Geometry check sheet. Reference: the model listing, model coordinates, mm. A direction names the side the tool comes from. Round coordinates to 2 decimals unless told otherwise and drop trailing zeros. Loops run counter-clockwise (first coordinate to the right, second up) from the corner with the lowest first, then second, coordinate; pieces in that order, holes last. Notation, with made-up numbers: (64, 45) - (111, 45) arc R8 cw to (111, 57) - close; hole circle Ø9 at (82, 41). An arc over 180 degrees is marked (long way). Answer as CSV lines item,"result". Start each with the question number.
1) Cross-section at A-A on z = 2.75. Record the boundary of the cut face in (x, y).
2) Cross-section at C-C on z = -0.5. Record the boundary of the cut face in (x, y) (3 decimals).
3) Cross-section at B-B on x = 0. Record the boundary of the cut face in (y, z), and give its area (3 significant figures).
4) Thickness scan on line 1 along Y through (x, z) = (0, 1.1); line 2 along Z through (x, y) = (9.75, -5.75); line 3 along X through (y, z) = (-5.5, -2.5). Record the ranges inside material, lowest first.
5) Draft check along Y on faces 1 (the cylindrical face through (-8.21, 8.65, 1.88)), 2 (the flat face through (0, -10.16, -2)), 3 (the cylindrical face through (-5.08, -0.13, 1.5)). Enter one of: released by +Y, released by -Y, zero draft, split by the parting line, or undercut.
6) Depth check by flat-ended pin: P1, Ø3, axis at x = -1.5, y = -2, coming from the +Z side. Enter the tip coordinate at first touch or a pass-through.
7) Cross-section at D-D on y = 0. Record the boundary of the cut face in (x, z).
8) Access from +Z, -Z, +X, -X, +Y, -Y to the whole of each face (thin tool, end or side, straight path). Record for faces 4 (the cylindrical face through (10.882, -0.101, -1.503)), 5 (the cylindrical face through (7.034, -6.493, 1.878)).
from build123d import *

# Parameters (mm, degrees)
BOSS_EXTRUDE5_DEPTH = 3.048
BOSS_EXTRUDE6_DEPTH = 3.048
PRONGS_R            = 1.27
BOSS_EXTRUDE7_DEPTH = 3.81


with BuildPart() as part:
    # Back Plate → Boss-Extrude5 (new body)
    with BuildSketch(Plane.XY):
        with BuildLine():
            Line((0, -10.16), (7.62, -10.16))
            ThreePointArc((7.62, -10.16), (9.416051224, -9.416051224), (10.16, -7.62))
            ThreePointArc((10.16, -7.62), (9.867513929, -5.715), (10.16, -3.81))
            ThreePointArc((10.16, -3.81), (10.882617987, -0.046833682), (10.16, 3.716332637))
            ThreePointArc((10.16, 3.716332637), (9.867513929, 5.621332637), (10.16, 7.526332637))
            ThreePointArc((10.16, 7.526332637), (9.416051224, 9.322383861), (7.62, 10.066332637))
            Line((7.62, 10.066332637), (-7.62, 10.066332637))
            ThreePointArc((-7.62, 10.066332637), (-9.416051224, 9.322383861), (-10.16, 7.526332637))
            ThreePointArc((-10.16, 7.526332637), (-9.867513929, 5.621332637), (-10.16, 3.716332637))
            ThreePointArc((-10.16, 3.716332637), (-10.882617987, -0.046833682), (-10.16, -3.81))
            ThreePointArc((-10.16, -3.81), (-9.867513929, -5.715), (-10.16, -7.62))
            ThreePointArc((-10.16, -7.62), (-9.416051224, -9.416051224), (-7.62, -10.16))
            Line((-7.62, -10.16), (0, -10.16))
        make_face()
    extrude(amount=-BOSS_EXTRUDE5_DEPTH)

    # Inner Circle → Boss-Extrude6 (add)
    with BuildSketch(Plane.XY):
        with BuildLine():
            Line((3.624386403, 3.559525699), (3.984498069, 3.917846237))
            ThreePointArc((3.984498069, 3.917846237), (-5.58790138, 0.033198873), (3.937664969, -3.96491344))
            Line((3.937664969, -3.96491344), (3.577553303, -3.606592902))
            ThreePointArc((3.577553303, -3.606592902), (-5.079891518, 0.033198873), (3.624386403, 3.559525699))
        make_face()
    extrude(amount=BOSS_EXTRUDE6_DEPTH)

    # Prongs → Boss-Extrude7 (add)
    with BuildSketch(Plane.XY):
        with Locations(Location((-7.62, 7.526332637, 0), (0, 0, 180))):
            Circle(PRONGS_R)
        with Locations(Location((7.62, -7.62, 0), (0, 0, 180))):
            Circle(PRONGS_R)
    extrude(amount=BOSS_EXTRUDE7_DEPTH)


solid = part.part
Answer block:
1,outline,"circle Ø2.54 at (-7.62, 7.53); (3.58, -3.61) arc R5.08 cw (long way) to (3.62, 3.56) - (3.98, 3.92) arc R5.59 ccw (long way) to (3.94, -3.96) - close; circle Ø2.54 at (7.62, -7.62)"
2,outline,"(-10.16, -7.62) arc R2.54 ccw to (-7.62, -10.16) - (7.62, -10.16) arc R2.54 ccw to (10.16, -7.62) arc R6.35 cw to (10.16, -3.81) arc R10.16 ccw to (10.16, 3.716) arc R6.35 cw to (10.16, 7.526) arc R2.54 ccw to (7.62, 10.066) - (-7.62, 10.066) arc R2.54 ccw to (-10.16, 7.526) arc R6.35 cw to (-10.16, 3.716) arc R10.16 ccw to (-10.16, -3.81) arc R6.35 cw to start"
3,outline,"(-10.16, -3.05) - (10.07, -3.05) - (10.07, 0) - (5.59, 0) - (5.59, 3.05) - (5.08, 3.05) - (5.08, 0) - (-5.08, 0) - (-5.08, 3.05) - (-5.59, 3.05) - (-5.59, 0) - (-10.16, 0) - close"
3,area,"64.7 mm^2"
4,line 1,"y = -5.59 to -5.08, 5.08 to 5.59"
4,line 2,"z = -3.05 to 0"
4,line 3,"x = -9.87 to 9.87"
5,face 1,"split by the parting line"
5,face 2,"released by -Y"
5,face 3,"undercut"
6,P1,"stops at z = 0"
7,outline,"(-10.88, -3.05) - (10.88, -3.05) - (10.88, 0) - (-5.08, 0) - (-5.08, 3.05) - (-5.59, 3.05) - (-5.59, 0) - (-10.88, 0) - close"
8,face 4,"+Z, -Z, +X"
8,face 5,"+Z"
